Autodesk Inventor part; units mm, degrees
ref_plane "YZ Plane" through (0, 0, 0) normal (1, 0, 0) x (0, 1, 0)
ref_plane "XZ Plane" through (0, 0, 0) normal (0, 1, 0) x (-1, 0, 0)
ref_plane "XY Plane" through (0, 0, 0) normal (0, 0, 1) x (1, 0, 0)
sketch "Sketch1" plane through (0, 0, 0) normal (0, 0, 1) x (1, 0, 0)
  line L0 (0, 0) -> (170.5, 0)
  line L1 (170.5, 0) -> (170.5, 86)
  line L2 (170.5, 86) -> (0, 86)
  line L3 (0, 86) -> (0, 0)
  line L4 (5, 5) -> (165.5, 5)
  line L5 (165.5, 5) -> (165.5, 81)
  line L6 (165.5, 81) -> (5, 81)
  line L7 (5, 81) -> (5, 5)
  line L8 (5, 81) -> (5, 86)
  line L9 (165.5, 81) -> (165.5, 86)
  dimension "d0" = 170.5
  dimension "d1" = 86
  dimension "d2" = 5
extrude "Extrusion1" add sketch "Sketch1" along normal blind 4 contours L3 L2 L8 L7 L4 L5 L9 L1 L0
sketch "Sketch2" plane through (0, 0, 0) normal (0, -1, 0) x (1, 0, 0)
  line L0 (0, 0) -> (170.5, 0) construction
  line L1 (170.5, 0) -> (0, 0) construction
  line L2 (0, 0) -> (0, -6) construction
  line L3 (0, -6) -> (170.5, -6) construction
  line L4 (170.5, -6) -> (170.5, 0) construction
  line L5 (170.5, -6) -> (0, -6) construction
  line L6 (0, -6) -> (0, 164.5) construction
  line L7 (0, 164.5) -> (170.5, 164.5) construction
  line L8 (170.5, 164.5) -> (170.5, -6) construction
  line L9 (170.5, -6) -> (0, -6)
  line L10 (0, -6) -> (0, 164.5)
  line L11 (0, 164.5) -> (170.5, 164.5)
  line L12 (170.5, 164.5) -> (170.5, -6)
  dimension "d5" = 6
  dimension "d6" = 170.5
  dimension "d7" = 170.5
extrude "Extrusion2" add sketch "Sketch2" along normal blind 2
sketch "Sketch3" plane through (170.5, 0, -6) normal (0, 0, -1) x (-1, 0, 0)
  line L0 (0, 86) -> (5, 86)
  line L1 (0, 0) -> (0, 86)
  line L2 (170.5, 0) -> (0, 0)
  line L3 (170.5, 86) -> (170.5, 0)
  line L4 (165.5, 86) -> (170.5, 86)
  line L5 (165.5, 5) -> (165.5, 86)
  line L6 (5, 5) -> (165.5, 5)
  line L7 (5, 86) -> (5, 5)
extrude "Extrusion3" add sketch "Sketch3" against normal blind 3.2
sketch "Sketch4" plane through (0, 0, 0) normal (-1, 0, 0) x (0, 0, 1)
  line L0 (0, 86) -> (0, 0) construction
  line L1 (4, 86) -> (4, 0) construction
  line L2 (0, 86) -> (4, 86) construction
  line L3 (-6, 86) -> (164.5, 86)
  line L4 (164.5, 86) -> (164.5, -2)
  line L5 (164.5, -2) -> (-6, -2)
  line L6 (-6, -2) -> (-6, 86)
  line L7 (0, 0) -> (-2.8, 0)
  line L8 (-2.8, 86) -> (-2.8, 0)
  line L9 (-6, 86) -> (-2.8, 86)
  line L10 (-6, 86) -> (-6, -2)
  line L11 (164.5, -2) -> (-6, -2)
  line L12 (164.5, 0) -> (164.5, -2)
  line L13 (164.5, 0) -> (4, 0)
extrude "Extrusion4" add sketch "Sketch4" along normal blind 3
sketch "Sketch5" plane through (170.5, 0, 0) normal (1, 0, 0) x (0, 0, -1)
  line L0 (6, -2) -> (-164.5, -2)
  line L1 (-164.5, 86) -> (-4, 86)
  line L2 (6, -2) -> (-164.5, -2)
  line L3 (-164.5, -2) -> (-164.5, 86)
  line L4 (-164.5, 86) -> (6, 86)
  line L5 (6, 86) -> (6, -2)
  point P0 (0, 0)
  point P1 (-4, 86)
extrude "Extrusion5" add sketch "Sketch5" along normal blind 3
sketch "Sketch6" plane through (0, 0, 164.5) normal (0, 0, 1) x (1, 0, 0)
  line L0 (-3, -2) -> (-3, 86)
  line L1 (173.5, 86) -> (173.5, -2)
  line L2 (-3, -2) -> (173.5, -2)
  line L3 (173.5, -2) -> (173.5, 86)
  line L4 (173.5, 86) -> (-3, 86)
  line L5 (-3, 86) -> (-3, -2)
  point P0 (0, 0)
  point P1 (173.5, -2)
  point P2 (-3, 86)
extrude "Extrusion6" add sketch "Sketch6" along normal blind 3
properties part number "Box"
Here's how the part is built. I have some questions about the finished solid (model axes, mm). A direction names the side the tool comes from. Round coordinates to 2 decimals unless told otherwise and drop trailing zeros. Order: outer loops, then holes, each group sorted by start corner. A loop starts at its lowest first (then second) coordinate and runs counter-clockwise, first axis right, second up. Notation, with made-up numbers: M 84,89.25 L 112,89.25 A24 cw 112,102.25 Z; hole C -26.75,-19 d8. An arc over 180 degrees is marked long. One line per question, with ' | ' between items.
1) I want a section at C-C, the plane z = 14. Write out the boundary of the cut face in (x, y).
Working result:
outline: M -3,-2 L 173.5,-2 L 173.5,86 L 170.5,86 L 170.5,0 L 0,0 L 0,86 L -3,86 Z
2) For faces 5 (the face through (79, 2, 4)), 6 (the face through (165.5, 45, 2)), 7 (the face through (173.5, 43, 80)), which set-ups out of +Z, -Z, +X, -X, +Y, -Y let a thin tool reach every point of the face, with its end or its side?
Working result:
face 5: +Y | face 6: -Z, +Y | face 7: +Z, -Z, +X, +Y, -Y
3) For pin 1 Ø4.5 at (x, z) = (56, 1.5) entering from +Y; pin 2 Ø0.8 at (x, z) = (115, -1.5) entering from +Y, each with a flat end and sliding along its axis, tell me the tip position at first contact or that it passes through.
Working result:
pin 1: y = 5 | pin 2: y = 0
4) If we mould it in two halves opening along X, with no side actions, what happens to faces 1 (the face through (0, 44, 83)), 2 (the face through (-3, 41, 80)), 3 (the face through (84, 43, 167.5)), 4 (the face through (92, 2, -2.8))? For each: +X half, -X half, draft (parallel to the pull), parting line (faces both ways), or undercut.
Working result:
face 1: undercut | face 2: -X half | face 3: draft | face 4: undercut
5) I need wall thicknesses on line 1 along X through (y, z) = (78, 104); line 2 along Z through (x, y) = (166, 50); line 3 along Z through (x, y) = (95.5, 33). Which ranges of each line are inside material? Lowest first, please.
Working result:
line 1: -3 to 0, 170.5 to 173.5 | line 2: -6 to -2.8, 0 to 4, 164.5 to 167.5 | line 3: 164.5 to 167.5
6) I want a section at B-B, the plane x = 123.5. Write out the boundary of the cut face in (y, z), then the cut area to 3 significant figures.
Working result:
outline: M -2,-6 L 5,-6 L 5,-2.8 L 0,-2.8 L 0,0 L 5,0 L 5,4 L 0,4 L 0,164.5 L 86,164.5 L 86,167.5 L -2,167.5 Z | area: 641 mm²
7) I want a section at A-A, the plane y = 45.5. Write out the boundary of the cut face in (x, z).
Working result:
outline: M -3,-6 L 5,-6 L 5,-2.8 L 0,-2.8 L 0,0 L 5,0 L 5,4 L 0,4 L 0,164.5 L 170.5,164.5 L 170.5,4 L 165.5,4 L 165.5,0 L 170.5,0 L 170.5,-2.8 L 165.5,-2.8 L 165.5,-6 L 173.5,-6 L 173.5,167.5 L -3,167.5 Z
